Verification items for the finished model (mm, model axes). A direction names the side the tool comes from. Coordinates: 2 decimals unless noted, no trailing zeros. Order: outer loops, then holes, each group sorted by start corner. A loop starts at its lowest first (then second) coordinate and runs counter-clockwise, first axis right, second up. Notation, with made-up numbers: M 19,-13 L 35,-13 A34 ccw 35,25 Z; hole C 57.25,87.25 d7. An arc over 180 degrees is marked long. Use one line per item in the form item = value. Start each with the question number.
```python
from build123d import *

# Parameters (mm, degrees)
F1_DEPTH = 12.7
F2_F1_R  = 1.27
F2_F2_R  = 1.27


with BuildPart() as f1:
    # F0 (on Right) → F1 (new body, symmetric)
    with BuildSketch(Plane.YZ):
        with BuildLine():
            ThreePointArc((-22.86, -11.0716033166), (-25.3986752482, 0.259414025), (-22.6290909091, 11.5362144843))
            Line((-22.6290909091, 11.5362144843), (-22.6290909091, 25.197786356))
            Line((-22.6290909091, 25.197786356), (-27.7090909091, 25.197786356))
            Line((-27.7090909091, 25.197786356), (-27.7090909091, 12.6979006529))
            ThreePointArc((-27.7090909091, 12.6979006529), (-30.48, 0), (-27.7090909091, -12.6979006529))
            Line((-27.7090909091, -12.6979006529), (-27.7090909091, -63.5))
            Line((-27.7090909091, -63.5), (-22.86, -63.5))
            Line((-22.86, -63.5), (22.86, -63.5))
            Line((22.86, -63.5), (27.7090909091, -63.5))
            Line((27.7090909091, -63.5), (27.7090909091, -12.6979006529))
            ThreePointArc((27.7090909091, -12.6979006529), (30.48, 0), (27.7090909091, 12.6979006529))
            Line((27.7090909091, 12.6979006529), (27.7090909091, 25.197786356))
            Line((27.7090909091, 25.197786356), (22.6290909091, 25.197786356))
            Line((22.6290909091, 25.197786356), (22.6290909091, 11.5362144843))
            ThreePointArc((22.6290909091, 11.5362144843), (25.3986752482, 0.259414025), (22.86, -11.0716033166))
            ThreePointArc((22.86, -11.0716033166), (0, -25.4), (-22.86, -11.0716033166))
        make_face()
    extrude(amount=F1_DEPTH, both=True)

    # F2: fillet of radius 1.27 on 31 edges, made by hand

    # F2_f1
    f2_f1_edges = [f1.edges().sort_by_distance(p)[0] for p in [
        (0, 27.7090909091, 12.6979006529),
        (0, 27.7090909091, -12.6979006529),
        (0, -27.7090909091, 12.6979006529),
        (0, -27.7090909091, -12.6979006529),
    ]]
    fillet(f2_f1_edges, radius=F2_F1_R)

    # F2_f2
    f2_f2_edges = [f1.edges().sort_by_distance(p)[0] for p in [
        (0, -22.6290909091, 25.197786356),
        (0, -27.7090909091, 25.197786356),
        (-12.7, -25.1690909091, 25.197786356),
        (12.7, -25.1690909091, 25.197786356),
        (12.7, 25.1690909091, 25.197786356),
        (-12.7, 25.1690909091, 25.197786356),
        (0, 22.6290909091, 25.197786356),
        (-6.35, -22.6290909091, 11.5362144843),
        (6.35, -22.6290909091, 11.5362144843),
        (-6.35, 22.6290909091, 11.5362144843),
        (6.35, 22.6290909091, 11.5362144843),
        (-12.7, -27.7090909091, -38.2360386617),
        (-12.7, 27.7090909091, 19.0849318397),
        (-12.7, 22.6290909091, 18.3670004202),
        (-12.7, 25.3986752482, 0.259414025),
        (-12.7, 0, -25.4),
        (-12.7, -25.3986752482, 0.259414025),
        (-12.7, -22.6290909091, 18.3670004202),
        (-12.7, -27.7090909091, 19.0849318397),
        (-12.7, -30.48, 0),
        (-12.7, 0, -63.5),
        (-12.7, 27.7090909091, -38.2360386617),
        (-12.7, 30.48, 0),
        (12.7, -30.48, 0),
        (12.7, 0, -25.4),
        (12.7, 30.48, 0),
        (12.7, 22.6290909091, 18.3670004202),
        (12.7, 25.3986752482, 0.259414025),
        (12.7, -25.3986752482, 0.259414025),
        (12.7, 27.7371090618, -12.7067829757),
        (12.7, 27.7371090618, 12.7067829757),
        (12.7, -27.7371090618, 12.7067829757),
        (12.7, -27.7371090618, -12.7067829757),
        (-12.7, 27.7371090618, -12.7067829757),
        (-12.7, 27.7371090618, 12.7067829757),
        (-12.7, -27.7371090618, 12.7067829757),
        (-12.7, -27.7371090618, -12.7067829757),
    ]]
    fillet(f2_f2_edges, radius=F2_F2_R)


solid = f1.part
```
1. Cross-section at A-A on z = -38. Enter the section's corners in (x, y).
2. Depth check by flat-ended pin: P1, Ø5, axis at x = 6, y = 20, coming from the +Z side; P2, Ø13.5, axis at x = -2, z = 20, coming from the +Y side; P3, Ø4, axis at x = 4.5, y = 10.5, coming from the +Z side. Enter the tip coordinate at first touch or a pass-through.
3. Tool access check on faces 1 (the flat face through (0, 27.709, -39)), 2 (the flat face through (0, 22.629, 18)), 3 (the flat face through (1, 0, -63.5)), 4 (the flat face through (0, -27.709, 19)). Record the directions out of +Z, -Z, +X, -X, +Y, -Y that give a thin tool (end or side, any length) a straight path to the whole face; none if there is none.
4. Material ranges on line 1 along Y through (x, z) = (0.25, 0); line 2 along Y through (x, z) = (4.5, -57); line 3 along Z through (x, y) = (2.5, 0), recorded low to high.
5. Release check for a two-part mould opening along Y. For faces 5 (the flat face through (0, 27.709, 19)), 6 (the flat face through (0, -27.709, -38)), 7 (the cylindrical face through (0.16, 0.72, -25.39)) record: pulls with the +Y half, pulls with the -Y half, needs draft (parallel to the pull), parting line crosses it, or undercut.
6. Cross-section at B-B on x = -6.25. Enter the section's corners in (y, z), and give its area (3 significant figures).
Final values:
q1.outline = M -12.7,-26.44 A1.27 ccw -11.43,-27.71 L 11.43,-27.71 A1.27 ccw 12.7,-26.44 L 12.7,26.44 A1.27 ccw 11.43,27.71 L -11.43,27.71 A1.27 ccw -12.7,26.44 Z
q2.P1 = -11.79
q2.P2 = 27.71
q2.P3 = -22.11
q3.face_1 = -Z, +X, -X, +Y
q3.face_2 = +Z, +X, -X
q3.face_3 = -Z, +X, -X, +Y, -Y
q3.face_4 = +Z, +X, -X, -Y
q4.line_1 = -30.48 to -25.4, 25.4 to 30.48
q4.line_2 = -27.71 to 27.71
q4.line_3 = -63.5 to -25.4
q5.face_5 = pulls with the +Y half
q5.face_6 = pulls with the -Y half
q5.face_7 = undercut
q6.outline = M -27.82,-12.45 A1.27 cw -27.71,-12.97 L -27.71,-63.5 L 27.71,-63.5 L 27.71,-12.97 A1.27 cw 27.82,-12.45 A30.48 ccw 27.82,12.45 A1.27 cw 27.71,12.97 L 27.71,25.2 L 23.9,25.2 A1.27 ccw 22.63,23.93 L 22.63,11.84 A1.27 ccw 22.76,11.27 A25.4 cw long -22.76,11.27 A1.27 ccw -22.63,11.84 L -22.63,23.93 A1.27 ccw -23.9,25.2 L -26.44,25.2 A1.27 ccw -27.71,23.93 L -27.71,12.97 A1.27 cw -27.82,12.45 A30.48 ccw Z
q6.area = 2,810 mm2
